Part model, mm, in its own coordinate system. Round coordinates to 2 decimals unless told otherwise and drop trailing zeros. Order: outer loops, then holes, each group sorted by start corner. A loop starts at its lowest first (then second) coordinate and runs counter-clockwise, first axis right, second up. Notation, with made-up numbers: (80.5, 10) - (117.5, 10) arc R30 cw to (117.5, 33) - close; hole circle Ø6 at (-36, 74). An arc over 180 degrees is marked (long way). Return JSON: item names as keys, results as strings. Group by question number.
Item 1: Two-plate mould, pull along Z, no slides. Class faces 1 (the face through (-831, 9, -190)), 2 (the face through (-444, 9, 0)), 3 (the face through (-444, 18.55, -29)): released by +Z, released by -Z, zero draft, split by the parting line, or undercut.
Item 2: Saw through at B-B on x = -839. List the corners of the cut face in (y, z), and give its area (3 significant figures).
Item 3: Saw through at D-D on x = -626. List the corners of the cut face in (y, z).
Item 4: Saw through at A-A on z = -200.5. List the corners of the cut face in (x, y), and give its area (3 significant figures).
Item 5: Saw through at C-C on z = -427. List the corners of the cut face in (x, y), and give its area (3 significant figures).
Item 6: Probe probe 1 along X at (y, z) = (5.75, -169); probe 2 along Z at (x, y) = (-175.5, 4); probe 3 along X at (y, z) = (7, -145). List the from-to ranges inside material, lowest first.
Autodesk Inventor part; units mm, degrees
ref_plane "YZ Plane" through (0, 0, 0) normal (1, 0, 0) x (0, 1, 0)
ref_plane "XZ Plane" through (0, 0, 0) normal (0, 1, 0) x (-1, 0, 0)
ref_plane "XY Plane" through (0, 0, 0) normal (0, 0, 1) x (1, 0, 0)
sketch "Sketch1" plane through (0, 0, 0) normal (0, 1, 0) x (-1, 0, 0)
  line L0 (0, 0) -> (900, 0)
  line L1 (900, 0) -> (900, -600)
  line L2 (900, -600) -> (0, -600)
  line L3 (0, -600) -> (0, 0)
  line L4 (725, -75) -> (175, -75)
  line L5 (175, -75) -> (175, -535)
  line L6 (175, -535) -> (725, -535)
  line L7 (725, -535) -> (725, -75)
  dimension "d0" = 900
  dimension "d1" = 600
  dimension "d23" = 175
  dimension "d24" = 75
  dimension "d25" = 460
  dimension "d26" = 550
extrude "Extrusion4" add sketch "Sketch1" along normal blind 18.55
sketch "Sketch4" plane through (0, 18.55, 0) normal (0, 1, 0) x (1, 0, 0)
  line L0 (-850, 440) -> (-812.9, 440)
  line L1 (-812.9, 440) -> (-812.9, 410)
  line L2 (-812.9, 410) -> (-850, 410)
  line L3 (-850, 410) -> (-850, 440)
  line L4 (-850, 160) -> (-812.9, 160)
  line L5 (-812.9, 160) -> (-812.9, 190)
  line L6 (-812.9, 190) -> (-850, 190)
  line L7 (-850, 190) -> (-850, 160)
  line L8 (-87.1, 440) -> (-50, 440)
  line L9 (-50, 440) -> (-50, 410)
  line L10 (-50, 410) -> (-87.1, 410)
  line L11 (-87.1, 410) -> (-87.1, 440)
  line L12 (-87.1, 160) -> (-50, 160)
  line L13 (-50, 160) -> (-50, 190)
  line L14 (-50, 190) -> (-87.1, 190)
  line L15 (-87.1, 190) -> (-87.1, 160)
  line L16 (0, 600) -> (-900, 600)
  line L17 (-900, 600) -> (-900, 0)
  line L18 (-900, 0) -> (0, 0)
  line L19 (0, 0) -> (0, 600)
  dimension "d29" = 160
  dimension "d30" = 50
  dimension "d33" = 30
  dimension "d34" = 37.1
  dimension "d35" = 30
  dimension "d36" = 50
  dimension "d39" = 160
extrude "Extrusion5" cut sketch "Sketch4" against normal blind 50 contours L0 L1 L2 L3 | L7 L6 L5 L4 | L8 L9 L10 L11 | L15 L14 L13 L12
properties part number "Table_plate"
Filled in:
{
 "1": {"face 1": "undercut", "face 2": "released by +Z", "face 3": "zero draft"},
 "2": {"outline": "(0, -600) - (18.55, -600) - (18.55, -440) - (0, -440) - close; (0, -410) - (18.55, -410) - (18.55, -190) - (0, -190) - close; (0, -160) - (18.55, -160) - (18.55, 0) - (0, 0) - close", "area": "10,000 mm^2"},
 "3": {"outline": "(0, -600) - (18.55, -600) - (18.55, -535) - (0, -535) - close; (0, -75) - (18.55, -75) - (18.55, 0) - (0, 0) - close"},
 "4": {"outline": "(-900, 0) - (-725, 0) - (-725, 18.55) - (-900, 18.55) - close; (-175, 0) - (0, 0) - (0, 18.55) - (-175, 18.55) - close", "area": "6,490 mm^2"},
 "5": {"outline": "(-900, 0) - (-850, 0) - (-850, 18.55) - (-900, 18.55) - close; (-812.9, 0) - (-725, 0) - (-725, 18.55) - (-812.9, 18.55) - close; (-175, 0) - (-87.1, 0) - (-87.1, 18.55) - (-175, 18.55) - close; (-50, 0) - (0, 0) - (0, 18.55) - (-50, 18.55) - close", "area": "5,120 mm^2"},
 "6": {"probe 1": "x = -900 to -850, -812.9 to -725, -175 to -87.1, -50 to 0", "probe 2": "z = -600 to -535, -75 to 0", "probe 3": "x = -900 to -725, -175 to 0"}
}
